Verification items for the finished model (mm, model axes). A direction names the side the tool comes from. Give positions to 0.01 mm unless a question says otherwise; leave off trailing zeros. Order: outer loops, then holes, each group sorted by start corner. A loop starts at its lowest first (then second) coordinate and runs counter-clockwise, first axis right, second up. Notation, with made-up numbers: M 75,18 L 108,18 A3 ccw 108,22 Z; hole C 62.25,-2 d9. An arc over 180 degrees is marked long. Answer as a JSON object with one key per item and string values.
```python
from build123d import *

# Parameters (mm, degrees)
SKETCH1_W           = 80.01
SKETCH1_H           = 36.068
BOSS_EXTRUDE1_DEPTH = 1.524
CUT_EXTRUDE1_REACH  = 45.908
SKETCH2_R           = 1.3335
SKETCH3_W           = 71.12
SKETCH3_H           = 24.13
BOSS_EXTRUDE2_DEPTH = 8.89
SKETCH4_W           = 2.921
SKETCH4_H           = 18.0848
BOSS_EXTRUDE3_DEPTH = 3.175


with BuildPart() as part:
    # Sketch1 → Boss-Extrude1 (new body)
    with BuildSketch(Plane(origin=(0, 0, 0), x_dir=(1, 0, 0), z_dir=(0, 1, 0))):
        Rectangle(SKETCH1_W, SKETCH1_H)
    extrude(amount=BOSS_EXTRUDE1_DEPTH)

    # Sketch2 → Cut-Extrude1 (cut, up to next)
    with BuildSketch(Plane(origin=(0, 1.524, 0), x_dir=(1, 0, 0), z_dir=(0, 1, 0)), mode=Mode.PRIVATE) as cut_extrude1_sk1:
        with Locations(Location((-36.068, 14.097, 0), (0, 0, 270))):
            Circle(SKETCH2_R)
    cut_extrude1_tool1 = extrude(cut_extrude1_sk1.sketch, amount=-CUT_EXTRUDE1_REACH, mode=Mode.PRIVATE) & part.part
    # Sketch2 → Cut-Extrude1 (cut, up to next)
    with BuildSketch(Plane(origin=(0, 1.524, 0), x_dir=(1, 0, 0), z_dir=(0, 1, 0)), mode=Mode.PRIVATE) as cut_extrude1_sk2:
        with Locations(Location((36.068, 14.097, 0), (0, 0, 270))):
            Circle(SKETCH2_R)
    cut_extrude1_tool2 = extrude(cut_extrude1_sk2.sketch, amount=-CUT_EXTRUDE1_REACH, mode=Mode.PRIVATE) & part.part
    # Sketch2 → Cut-Extrude1 (cut, up to next)
    with BuildSketch(Plane(origin=(0, 1.524, 0), x_dir=(1, 0, 0), z_dir=(0, 1, 0)), mode=Mode.PRIVATE) as cut_extrude1_sk3:
        with Locations(Location((36.068, -14.097, 0), (0, 0, 270))):
            Circle(SKETCH2_R)
    cut_extrude1_tool3 = extrude(cut_extrude1_sk3.sketch, amount=-CUT_EXTRUDE1_REACH, mode=Mode.PRIVATE) & part.part
    # Sketch2 → Cut-Extrude1 (cut, up to next)
    with BuildSketch(Plane(origin=(0, 1.524, 0), x_dir=(1, 0, 0), z_dir=(0, 1, 0)), mode=Mode.PRIVATE) as cut_extrude1_sk4:
        with Locations(Location((-36.068, -14.097, 0), (0, 0, 270))):
            Circle(SKETCH2_R)
    cut_extrude1_tool4 = extrude(cut_extrude1_sk4.sketch, amount=-CUT_EXTRUDE1_REACH, mode=Mode.PRIVATE) & part.part
    add(cut_extrude1_tool1.solids().sort_by_distance((-36.068, 1.524, -14.097))[0], mode=Mode.SUBTRACT)
    add(cut_extrude1_tool2.solids().sort_by_distance((36.068, 1.524, -14.097))[0], mode=Mode.SUBTRACT)
    add(cut_extrude1_tool3.solids().sort_by_distance((36.068, 1.524, 14.097))[0], mode=Mode.SUBTRACT)
    add(cut_extrude1_tool4.solids().sort_by_distance((-36.068, 1.524, 14.097))[0], mode=Mode.SUBTRACT)

    # Sketch3 → Boss-Extrude2 (add)
    with BuildSketch(Plane(origin=(0, 1.524, 0), x_dir=(1, 0, 0), z_dir=(0, 1, 0))):
        Rectangle(SKETCH3_W, SKETCH3_H)
    extrude(amount=BOSS_EXTRUDE2_DEPTH)

    # Sketch4 → Boss-Extrude3 (add)
    with BuildSketch(Plane(origin=(0, 1.524, 0), x_dir=(1, 0, 0), z_dir=(0, 1, 0))):
        with Locations((-37.0205, 0.0254)):
            Rectangle(SKETCH4_W, SKETCH4_H)
    extrude(amount=BOSS_EXTRUDE3_DEPTH)


solid = part.part
```
Q1. Release check for a two-part mould opening along X. For faces 6 (the face through (-34.746, 0.773, -14.271)), 7 (the face through (0, 10.414, 0)), 8 (the face through (35.56, 6, 0)) record: +X half, -X half, draft (parallel to the pull), parting line (faces both ways), or undercut.
Resolved:
{"face 6": "undercut", "face 7": "draft", "face 8": "+X half"}
Q2. Section check B-B on z = -14. Record the cut outline in (x, y) (3 decimals).
Resolved:
{"outline": "M -40.005,0 L -37.398,0 L -37.398,1.524 L -40.005,1.524 Z; M -34.738,0 L 34.738,0 L 34.738,1.524 L -34.738,1.524 Z; M 37.398,0 L 40.005,0 L 40.005,1.524 L 37.398,1.524 Z"}
Q3. Tool access check on faces 1 (the face through (-38.481, 3, 0)), 2 (the face through (0, 6, 12.065)), 3 (the face through (-37, 3, 9.017)), 4 (the face through (0, 6, -12.065)), 5 (the face through (-37, 3, -9.068)). Record the directions out of +Z, -Z, +X, -X, +Y, -Y that give a thin tool (end or side, any length) a straight path to the whole face; none if there is none.
Resolved:
{"face 1": "+Z, -Z, -X, +Y", "face 2": "+Z, +X, -X, +Y", "face 3": "+Z, -X, +Y", "face 4": "-Z, +X, -X, +Y", "face 5": "-Z, -X, +Y"}
Q4. Gauge pin test, flat ends, axial feed: pin 1 Ø5 at (x, y) = (-29, 5) entering from +Z (3 decimals); pin 2 Ø4.5 at (y, z) = (4, 4) entering from -X; pin 3 Ø2 at (x, z) = (-2, -14) entering from +Y; pin 4 Ø2 at (x, z) = (-36.068, -14.097) entering from +Y. Record the tip position at first contact, or that the pin passes through.
Resolved:
{"pin 1": "stops at z = 12.065", "pin 2": "stops at x = -38.48", "pin 3": "stops at y = 1.52", "pin 4": "passes through"}
Q5. Material ranges on L1, parallel to Y at x = 34, z = 14; L2, parallel to X at y = 9, z = 11; L3, parallel to X at y = 3, z = -3.5, recorded low to high.
Resolved:
{"L1": "y = 0 to 1.52", "L2": "x = -35.56 to 35.56", "L3": "x = -38.48 to 35.56"}
Q6. Section check C-C on x = 18.5. Record the cut outline in (y, z) (3 decimals).
Resolved:
{"outline": "M 0,-18.034 L 1.524,-18.034 L 1.524,-12.065 L 10.414,-12.065 L 10.414,12.065 L 1.524,12.065 L 1.524,18.034 L 0,18.034 Z"}
Q7. Section check A-A on y = 3. Record the cut outline in (x, z) (3 decimals), then the cut area to 3 significant figures.
Resolved:
{"outline": "M -38.481,-9.068 L -35.56,-9.068 L -35.56,-12.065 L 35.56,-12.065 L 35.56,12.065 L -35.56,12.065 L -35.56,9.017 L -38.481,9.017 Z", "area": "1,770 mm²"}
Q8. Section check D-D on z = -0.5. Record the cut outline in (x, y) (3 decimals), then the cut area to 3 significant figures.
Resolved:
{"outline": "M -40.005,0 L 40.005,0 L 40.005,1.524 L 35.56,1.524 L 35.56,10.414 L -35.56,10.414 L -35.56,4.699 L -38.481,4.699 L -38.481,1.524 L -40.005,1.524 Z", "area": "763 mm²"}
